Verification items for the finished model (mm, model axes). Face numbers are marked on the shaded views. A direction names the side the tool comes from. Give positions to 0.01 mm unless a question says otherwise; leave off trailing zeros. Write each loop counter-clockwise with the first axis right and the second up, starting at its lowest first coordinate (ties: lowest second). Pieces come first, ordered by that corner, then holes. Notation, with made-up numbers: (23.25, -17.5) -> (39.25, -17.5) arc R29 ccw to (39.25, 14.5) -> close; hole circle Ø3 at (-14.5, -9). An arc over 180 degrees is marked (long way). Answer as CSV lines item,"result". Start each with the question number.
1) Sectioned sample at B-B on z = -34. Record the cut outline in (x, y).
2) Material ranges on L1, parallel to X at y = 6.5, z = -22; L2, parallel to X at y = 20.5, z = -38; L3, parallel to Z at x = 96, y = 39, recorded low to high.
3) Tool access check on the marked faces 1, 2, 3, 4 and 5. Record the directions out of +Z, -Z, +X, -X, +Y, -Y that give a thin tool (end or side, any length) a straight path to the whole face; none if there is none.
4) Sectioned sample at C-C on z = -22. Record the cut outline in (x, y), and give its area (3 significant figures).
5) Mould release check, pull along X, two halves, no side actions. Record for the marked faces 6, 7 and 8: released by +X, released by -X, zero draft, split by the parting line, or undercut.
6) Sectioned sample at D-D on x = 80. Record the cut outline in (y, z).
7) Sectioned sample at A-A on y = 10.5. Record the cut outline in (x, z).
8) Gauge pin test, flat ends, axial feed: pin 1 Ø3 at (x, y) = (100.5, 5.5) entering from -Z; pin 2 Ø5 at (x, y) = (2.5, 7.5) entering from +Z; pin 3 Ø12 at (y, z) = (19.5, -40.5) entering from -X; pin 4 Ø5 at (x, z) = (96.5, -22) entering from -Y. Record the tip position at first contact, or that the pin passes through.
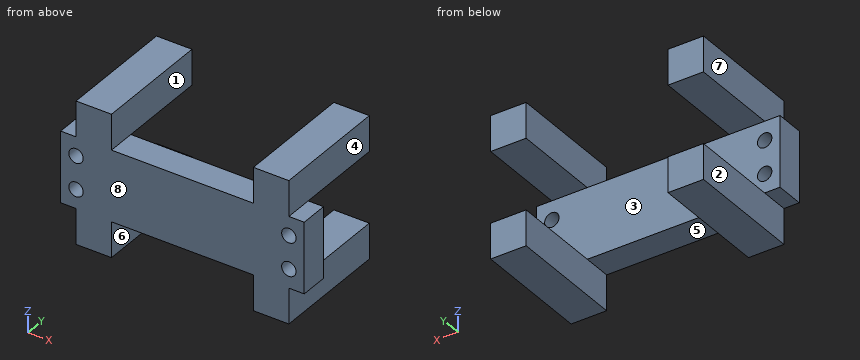
```python
from build123d import *

# Parameters (mm, degrees)
SKETCH1_W           = 103
SKETCH1_H           = 30
BOSS_EXTRUDE1_DEPTH = 12
SKETCH2_R           = 3.05
CUT_EXTRUDE1_DEPTH  = 12
SKETCH4_W           = 15
SKETCH4_H           = 15
BOSS_EXTRUDE3_DEPTH = 50


with BuildPart() as part:
    # Sketch1 → Boss-Extrude1 (new body)
    with BuildSketch(Plane(origin=(0, 0, 0), x_dir=(1, 0, 0), z_dir=(0, 1, 0))):
        with Locations((51.5, 15)):
            Rectangle(SKETCH1_W, SKETCH1_H)
    extrude(amount=BOSS_EXTRUDE1_DEPTH)

    # Sketch2 → Cut-Extrude1 (cut)
    with BuildSketch(Plane(origin=(0, 12, 0), x_dir=(1, 0, 0), z_dir=(0, 1, 0))):
        with Locations(Location((6.5, 8, 0), (0, 0, 270))):
            Circle(SKETCH2_R)
        with Locations(Location((6.5, 22, 0), (0, 0, 90))):
            Circle(SKETCH2_R)
        with Locations(Location((96.5, 8, 0), (0, 0, 90))):
            Circle(SKETCH2_R)
        with Locations(Location((96.5, 22, 0), (0, 0, 270))):
            Circle(SKETCH2_R)
    extrude(amount=-CUT_EXTRUDE1_DEPTH, mode=Mode.SUBTRACT)

    # Sketch4 → Boss-Extrude3 (add)
    with BuildSketch(Plane.XZ):
        with Locations((89, 7.5)):
            Rectangle(SKETCH4_W, SKETCH4_H)
        with Locations((89, -37.5)):
            Rectangle(SKETCH4_W, SKETCH4_H)
        with Locations((14, -37.5)):
            Rectangle(SKETCH4_W, SKETCH4_H)
        with Locations((14, 7.5)):
            Rectangle(SKETCH4_W, SKETCH4_H)
    extrude(amount=-BOSS_EXTRUDE3_DEPTH)


solid = part.part
```
Ans:
1,outline,"(6.5, 0) -> (21.5, 0) -> (21.5, 50) -> (6.5, 50) -> close; (81.5, 0) -> (96.5, 0) -> (96.5, 50) -> (81.5, 50) -> close"
2,L1,"x = 0 to 3.45, 9.55 to 93.45, 99.55 to 103"
2,L2,"x = 6.5 to 21.5, 81.5 to 96.5"
2,L3,"z = -45 to -30, 0 to 15"
3,face 1,"+Z, +Y, -Y"
3,face 2,"-Z, -X, +Y, -Y"
3,face 3,"+X, -X, +Y"
3,face 4,"+Z, +X, +Y, -Y"
3,face 5,"-Z, +Y, -Y"
4,outline,"(0, 0) -> (3.45, 0) -> (3.45, 12) -> (0, 12) -> close; (9.55, 0) -> (93.45, 0) -> (93.45, 12) -> (9.55, 12) -> close; (99.55, 0) -> (103, 0) -> (103, 12) -> (99.55, 12) -> close"
4,area,"1,090 mm²"
5,face 6,"undercut"
5,face 7,"released by -X"
5,face 8,"zero draft"
6,outline,"(0, -30) -> (12, -30) -> (12, 0) -> (0, 0) -> close"
7,outline,"(0, -30) -> (6.5, -30) -> (6.5, -45) -> (21.5, -45) -> (21.5, -30) -> (81.5, -30) -> (81.5, -45) -> (96.5, -45) -> (96.5, -30) -> (103, -30) -> (103, 0) -> (96.5, 0) -> (96.5, 15) -> (81.5, 15) -> (81.5, 0) -> (21.5, 0) -> (21.5, 15) -> (6.5, 15) -> (6.5, 0) -> (0, 0) -> close; hole circle Ø6.1 at (6.5, -22); hole circle Ø6.1 at (6.5, -8); hole circle Ø6.1 at (96.5, -22); hole circle Ø6.1 at (96.5, -8)"
8,pin 1,"stops at z = -30"
8,pin 2,"stops at z = 0"
8,pin 3,"stops at x = 6.5"
8,pin 4,"passes through"
